```python
from build123d import *

# Parameters (mm, degrees)
F0_W     = 12
F0_H     = 10
F1_DEPTH = 9
F3_DEPTH = 15
F5_DEPTH = 11


with BuildPart() as f1:
    # F0 (on Front) → F1 (new body)
    with BuildSketch(Plane.XZ):
        with Locations((6, 5)):
            Rectangle(F0_W, F0_H)
    extrude(amount=F1_DEPTH)

    # F2 (on face) → F3 (join)
    with BuildSketch(Plane(origin=(0, 0, 0), x_dir=(-1, 0, 0), z_dir=(0, 1, 0))):
        with BuildLine():
            Line((-2, 10), (-10, 10))
            add(Edge.make_bspline(
                [(-12, 5), (-12, 6.6666666667), (-11, 8.3333333333), (-10, 10)],
                knots=[0.5, 0.5, 0.5, 0.5, 1, 1, 1, 1], degree=3))
            add(Edge.make_bspline(
                [(-10, 0), (-11, 1.6666666667), (-12, 3.3333333333), (-12, 5)],
                knots=[0, 0, 0, 0, 0.5, 0.5, 0.5, 0.5], degree=3))
            Line((-10, 0), (-2, 0))
            add(Edge.make_bspline(
                [(0, 5), (0, 3.3333333333), (-1, 1.6666666667), (-2, 0)],
                knots=[0.5, 0.5, 0.5, 0.5, 1, 1, 1, 1], degree=3))
            add(Edge.make_bspline(
                [(-2, 10), (-1, 8.3333333333), (0, 6.6666666667), (0, 5)],
                knots=[0, 0, 0, 0, 0.5, 0.5, 0.5, 0.5], degree=3))
        make_face()
    extrude(amount=F3_DEPTH)

    # F4 (on face) → F5 (join)
    with BuildSketch(Plane.XZ.offset(9)):
        with BuildLine():
            Line((6, 6), (4.8819660113, 6))
            ThreePointArc((4.8819660113, 6), (6, 3.5), (7.1180339887, 6))
            Line((7.1180339887, 6), (6, 6))
        make_face()
    extrude(amount=F5_DEPTH)


solid = f1.part
```
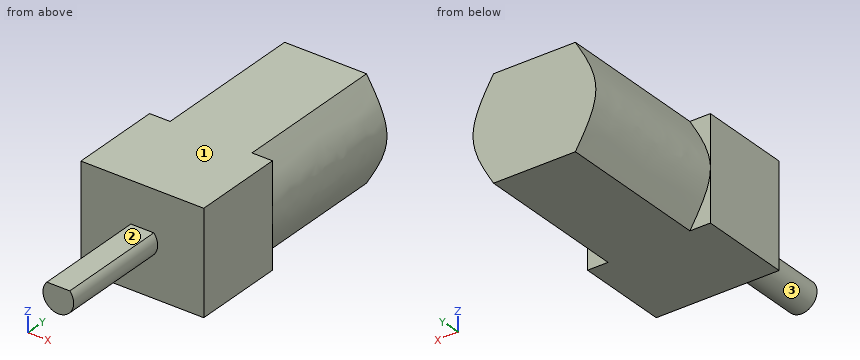
The listing builds one solid part. Answer for the finished solid, in the listing's coordinates (mm). Face numbers are marked on the shaded views. A direction names the side the tool comes from. Round coordinates to 2 decimals unless told otherwise and drop trailing zeros. Order: outer loops, then holes, each group sorted by start corner. A loop starts at its lowest first (then second) coordinate and runs counter-clockwise, first axis right, second up. Notation, with made-up numbers: (-28.5, -24) -> (17.5, -24) arc R33 cw to (17.5, 12) -> close; hole circle Ø2 at (-2, -23). An arc over 180 degrees is marked (long way). Answer as CSV lines item,"result".
Q1. Consider line 1 (Y direction, x = 7.25, z = 6); line 2 (X direction, y = 9.5, z = 1.75); line 3 (X direction, y = 10, z = 2.75). Determine where each line is inside the solid, lowest interval first. Write a range as from..to.
Computed values:
line 1,"y = -9..15"
line 2,"x = 0.99..11.01"
line 3,"x = 0.52..11.48"
Q2. A cutting plane is placed at B-B on y = -12. Determine the outline of the cut face in (x, z), plus the area to 3 significant figures.
Computed values:
outline,"(4.88, 6) arc R1.5 ccw (long way) to (7.12, 6) -> close"
area,"6.29 mm^2"
Q3. A cutting plane is placed at A-A on x = 6. Determine the outline of the cut face in (y, z).
Computed values:
outline,"(-20, 3.5) -> (-9, 3.5) -> (-9, 0) -> (15, 0) -> (15, 10) -> (-9, 10) -> (-9, 6) -> (-20, 6) -> close"
Q4. Which of the six approach directions +Z, -Z, +X, -X, +Y, -Y give full straight-line access (tool end or side, diameter ignored) to the marked faces 1, 2 and 3?
Computed values:
face 1,"+Z, +X, -X, +Y, -Y"
face 2,"+Z, +X, -X, -Y"
face 3,"-Y"
Q5. Given pin 1 (0.7 mm diameter, centred on x = 6, y = -12, fed in from +Z); pin 2 (1 mm diameter, centred on y = 11.5, z = 3, fed in from +X); pin 3 (1 mm diameter, centred on y = -13, z = 2.5, fed in from +X), each flat-ended and moving along its own axis, determine where each tip first touches the part or whether it passes through.
Computed values:
pin 1,"stops at z = 6"
pin 2,"stops at x = 11.76"
pin 3,"passes through"
